Study the drawing (mm; zero at the part's minimum x, y, z) and answer. A direction names the side the tool comes from. Round coordinates to 2 decimals unless told otherwise and drop trailing zeros. Order: outer loops, then holes, each group sorted by start corner. A loop starts at its lowest first (then second) coordinate and runs counter-clockwise, first axis right, second up. Notation, with made-up numbers: (1.5, 42) - (12.5, 42) arc R27 cw to (12.5, 75) - close; hole circle Ø1 at (45.25, 16.25). An arc over 180 degrees is marked (long way). Use one line per item in the form item = value. Start each with the question number.
Q1. The part is cut by section C-C on z = 33. Determine the outline of the cut face in (x, y), plus the area to 3 significant figures.
Q2. The part is cut by section A-A on y = 16. Determine the outline of the cut face in (x, z), plus the area to 3 significant figures.
Q3. Given P1, Ø4, axis at x = 20, y = 16, coming from the +Z side; P2, Ø8, axis at x = 17, z = 30, coming from the +Y side, each flat-ended and moving along its own axis, determine where each tip first touches the part or whether it passes through.
Q4. The part is cut by section D-D on x = 15. Determine the outline of the cut face in (y, z).
Q5. The part is cut by section B-B on x = 20. Determine the outline of the cut face in (y, z).
Q6. Find the intervals of material crossed by line 1 (Z direction, x = 35, y = 1.5); line 2 (Y direction, x = 20, z = 1.15); line 3 (Y direction, x = 5, z = 23), in increasing order. Write a range as [from, to].
Q7. Which of the six approach directions +Z, -Z, +X, -X, +Y, -Y give full straight-line access (tool end or side, diameter ignored) to the marked faces 1 and 2?
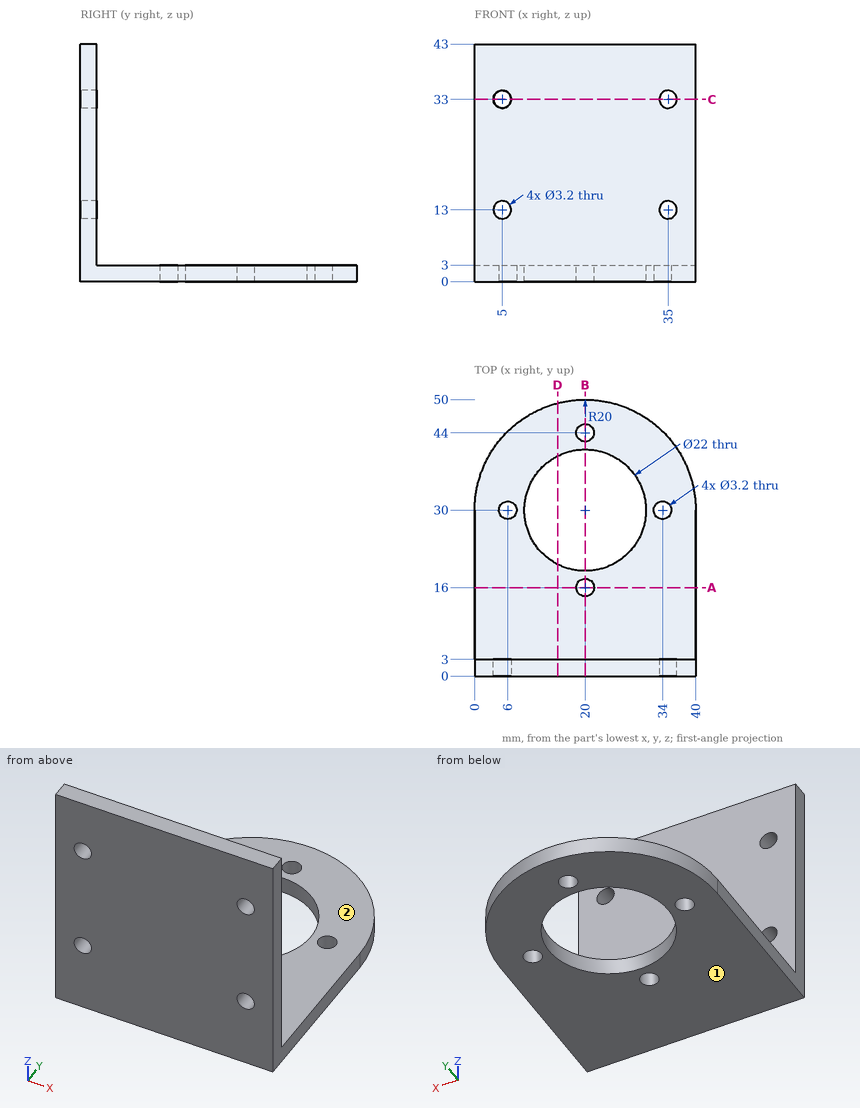
Found:
q1.outline = (0, 0) - (3.4, 0) - (3.4, 3) - (0, 3) - close; (6.6, 0) - (33.4, 0) - (33.4, 3) - (6.6, 3) - close; (36.6, 0) - (40, 0) - (40, 3) - (36.6, 3) - close
q1.area = 101 mm²
q2.outline = (0, 0) - (18.4, 0) - (18.4, 3) - (0, 3) - close; (21.6, 0) - (40, 0) - (40, 3) - (21.6, 3) - close
q2.area = 110 mm²
q3.P1 = 3
q3.P2 = 3
q4.outline = (0, 0) - (20.2, 0) - (20.2, 3) - (3, 3) - (3, 43) - (0, 43) - close; (39.8, 0) - (49.36, 0) - (49.36, 3) - (39.8, 3) - close
q5.outline = (0, 0) - (14.4, 0) - (14.4, 3) - (3, 3) - (3, 43) - (0, 43) - close; (17.6, 0) - (19, 0) - (19, 3) - (17.6, 3) - close; (41, 0) - (42.4, 0) - (42.4, 3) - (41, 3) - close; (45.6, 0) - (50, 0) - (50, 3) - (45.6, 3) - close
q6.line_1 = [0, 11.4], [14.6, 31.4], [34.6, 43]
q6.line_2 = [0, 14.4], [17.6, 19], [41, 42.4], [45.6, 50]
q6.line_3 = [0, 3]
q7.face_1 = -Z, +X, -X, +Y, -Y
q7.face_2 = +Z, +X, -X, +Y
